from build123d import *

# Parameters (mm, degrees)
SKETCH1_W           = 40
SKETCH1_H           = 51.6
BOSS_EXTRUDE1_DEPTH = 3
SKETCH2_W           = 28
SKETCH2_H           = 18
CUT_EXTRUDE1_DEPTH  = 66.357172521
CUT_EXTRUDE2_DEPTH  = 1
CUT_EXTRUDE2_DRAFT  = -60
CUT_EXTRUDE3_DEPTH  = 1
CUT_EXTRUDE3_DRAFT  = -60


with BuildPart() as part:
    # Sketch1 → Boss-Extrude1 (new body)
    with BuildSketch(Plane.XY):
        with Locations((20, 25.8)):
            Rectangle(SKETCH1_W, SKETCH1_H)
    extrude(amount=-BOSS_EXTRUDE1_DEPTH)

    # Sketch2 → Cut-Extrude1 (cut, through all)
    with BuildSketch(Plane(origin=(0, 0, -3), x_dir=(-1, 0, 0), z_dir=(0, 0, -1))):
        with Locations((-20, 25.8)):
            Rectangle(SKETCH2_W, SKETCH2_H)
    extrude(amount=-CUT_EXTRUDE1_DEPTH, mode=Mode.SUBTRACT)


with BuildPart() as cut_extrude2_tool:
    # Sketch3 → Cut-Extrude2 (with draft: the straight prism first)
    with BuildSketch(Plane.XY):
        with BuildLine():
            Line((35, 48.35), (30, 48.35))
            ThreePointArc((30, 48.35), (28.25, 46.6), (30, 44.85))
            Line((30, 44.85), (35, 44.85))
            ThreePointArc((35, 44.85), (36.75, 46.6), (35, 48.35))
        make_face()
    extrude(amount=-CUT_EXTRUDE2_DEPTH)
    # Cut-Extrude2: the draft: its side faces are tilted about the plane it starts from
    cut_extrude2_sides = [cut_extrude2_tool.faces().sort_by_distance(p)[0] for p in [
        (32.5, 48.35, -0.5),
        (28.25, 46.6, -0.5),
        (32.5, 44.85, -0.5),
        (36.75, 46.6, -0.5),
    ]]
    draft(cut_extrude2_sides, Plane.XY, CUT_EXTRUDE2_DRAFT)


with BuildPart() as part_1:
    add(part.part)

    # Cut-Extrude2: cut by cut_extrude2_tool
    add(cut_extrude2_tool.part, mode=Mode.SUBTRACT)


with BuildPart() as cut_extrude3_tool:
    # Sketch4 → Cut-Extrude3 (with draft: the straight prism first)
    with BuildSketch(Plane.XY):
        Polygon((15.669872981, 5), (22.165063509, 1.25), (22.165063509, 8.75), align=None)
    extrude(amount=-CUT_EXTRUDE3_DEPTH)
    # Cut-Extrude3: the draft: its side faces are tilted about the plane it starts from
    cut_extrude3_sides = [cut_extrude3_tool.faces().sort_by_distance(p)[0] for p in [
        (18.917468245, 3.125, -0.5),
        (22.165063509, 5, -0.5),
        (18.917468245, 6.875, -0.5),
    ]]
    draft(cut_extrude3_sides, Plane.XY, CUT_EXTRUDE3_DRAFT)


with BuildPart() as part_2:
    add(part_1.part)

    # Cut-Extrude3: cut by cut_extrude3_tool
    add(cut_extrude3_tool.part, mode=Mode.SUBTRACT)


solid = part_2.part
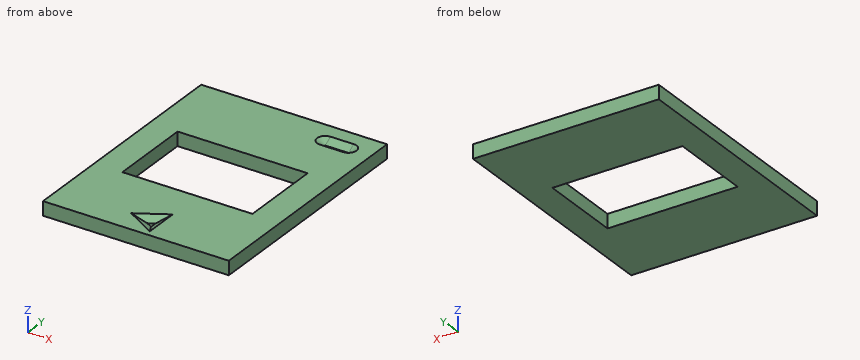
The listing builds one solid part. Answer for the finished solid, in the listing's coordinates (mm). Give positions to 0.01 mm unless a question says otherwise; leave off trailing zeros. Write each loop counter-clockwise with the first axis right and the second up, starting at its lowest first coordinate (ties: lowest second). Pieces come first, ordered by that corner, then holes.
1) Section A-A (y = 23) is taken. Write down the section's boundary in (x, z), and give its area (3 significant figures).
2) Section C-C (z = -2.1) is taken. Write down the section's boundary in (x, y).
3) Section D-D (x = 9.5) is taken. Write down the section's boundary in (y, z).
4) Given P1, Ø0.6, axis at x = 20, y = 5, coming from the +Z side, flat-ended and moving along its own axis, determine where the tip first touches the part or whether it passes through.
5) Find the intervals of material crossed by L1, parallel to Y at x = 27.5, z = -0.85; L2, parallel to Y at x = 31.5, z = -0.9; L3, parallel to X at y = 22, z = -1.5, in increasing order.
Response:
1. outline: (0, -3) - (6, -3) - (6, 0) - (0, 0) - close; (34, -3) - (40, -3) - (40, 0) - (34, 0) - close
1. area: 36.0 mm2
2. outline: (0, 0) - (40, 0) - (40, 51.6) - (0, 51.6) - close; hole (6, 16.8) - (34, 16.8) - (34, 34.8) - (6, 34.8) - close
3. outline: (0, -3) - (16.8, -3) - (16.8, 0) - (0, 0) - close; (34.8, -3) - (51.6, -3) - (51.6, 0) - (34.8, 0) - close
4. P1: stops at z = -1
5. L1: y = 0 to 16.8, 34.8 to 51.6
5. L2: y = 0 to 16.8, 34.8 to 46.41, 46.79 to 51.6
5. L3: x = 0 to 6, 34 to 40
